Model file for the job. Use its own axes, mm. A direction names the side the tool comes from. Coordinates: 2 decimals unless noted, no trailing zeros. Write each loop counter-clockwise with the first axis right and the second up, starting at its lowest first coordinate (ties: lowest second). Pieces come first, ordered by that corner, then holes. Notation, with made-up numbers: (-15, 58) -> (13, 58) arc R25 cw to (13, 76) -> close; hole circle Ø4 at (1, 63). An arc over 180 degrees is marked (long way). Answer as a JSON object with one key per item and string values. Group by question number.
from build123d import *

# Parameters (mm, degrees)
F1_DEPTH = 63.5
F2_DEPTH = 7.9375
F3_R     = 6.35
F4_DEPTH = 25.4


with BuildPart() as f1:
    # F0 (on Front) → F1 (new body, symmetric)
    with BuildSketch(Plane.XZ):
        Polygon((22.225, 9.525), (-41.275, 9.525), (-41.275, -9.525), (41.275, -9.525), (41.275, 9.525), align=None)
    extrude(amount=F1_DEPTH, both=True)

    # F0 (on Front) → F2 (join, symmetric)
    with BuildSketch(Plane.XZ):
        with BuildLine():
            add(Edge.make_bspline(
                [(-41.275, 9.525), (-41.231316, 40.761163), (-0.825848, 60.309073), (55.42913, 61.882778)],
                knots=[0, 0, 0, 0, 110.382184, 110.382184, 110.382184, 110.382184], degree=3))
            Line((-41.275, 9.525), (22.225, 9.525))
            Line((22.225, 9.525), (22.225, 27.0002))
            ThreePointArc((22.225, 27.0002), (31.853192, 51.0798), (55.42913, 61.882778))
        make_face()
    extrude(amount=F2_DEPTH, both=True)

    # F3
    f3_edges = [f1.edges().sort_by_distance(p)[0] for p in [
        (41.275, -63.5, 0),
        (-41.275, -63.5, 0),
        (41.275, 63.5, 0),
        (-41.275, 63.5, 0),
    ]]
    fillet(f3_edges, radius=F3_R)

    # F0 (on Front) → F4 (join, symmetric)
    with BuildSketch(Plane.XZ):
        with BuildLine():
            Line((22.225, 27.0002), (22.225, 9.525))
            Line((22.225, 9.525), (41.275, 9.525))
            Line((41.275, 9.525), (41.275, 27.0002))
            ThreePointArc((41.275, 27.0002), (45.92468, 38.22552), (57.15, 42.8752))
            Line((57.15, 42.8752), (60.325, 42.8752))
            Line((60.325, 42.8752), (60.325, 61.9252))
            Line((60.325, 61.9252), (57.15, 61.9252))
            add(Edge.make_bspline(
                [(55.42913, 61.882778), (56.001123, 61.898779), (56.574755, 61.912922), (57.15, 61.9252)],
                knots=[110.382184, 110.382184, 110.382184, 110.382184, 111.504536, 111.504536, 111.504536, 111.504536], degree=3))
            ThreePointArc((55.42913, 61.882778), (31.853192, 51.0798), (22.225, 27.0002))
        make_face()
        Polygon((60.325, 66.675), (60.325, 61.9252), (60.325, 42.8752), (85.435174, 42.8752), (85.435174, 66.675), align=None)
    extrude(amount=F4_DEPTH, both=True)

    # F0 (on Front) → F5 (revolve)
    with BuildSketch(Plane.XZ):
        Polygon((85.435174, 66.675), (85.435174, 42.8752), (85.435174, 38.1), (111.125, 38.1), (111.125, 66.675), align=None)
    revolve(axis=Axis((85.435174, 0, 52.3875), (0, 0, 1)))


solid = f1.part
(1) Pin check, flat tips, straight feed: pin 1 (2.5 mm diameter, centred on y = 12, z = 65.5, fed in from -X) (3 decimals); pin 2 (10 mm diameter, centred on y = -31.5, z = 5, fed in from +X) (3 decimals); pin 3 (6 mm diameter, centred on x = 80.5, z = 37.5, fed in from +Y); pin 4 (14 mm diameter, centred on y = -16.5, z = 14.5, fed in from -X) (3 decimals). Stop position of each tip, or through.
(2) Wall check: probe 1 along Y at (x, z) = (72.5, 52); probe 2 along X at (y, z) = (48, -0.5) (3 decimals); probe 3 along Z at (x, y) = (-31, 22.5) (3 decimals). Give the ranges that are in metal, low to high.
(3) Pull direction X, two halves, no side cores. Call faces 1 (the face through (-41.275, -1, 0)), 2 (the face through (0, 63.5, 0)), 3 (the face through (59, 2, 42.875)): released by +X, released by -X, zero draft, split by the parting line, or undercut.
(4) Cut at A-A on y = 43. List the corners of the cut face in (x, z) (3 decimals).
(5) 3-axis set-ups, long thin cutter, end or side, ignore diameter. For faces 4 (the face through (86, 0, 38.1)), 5 (the face through (51, 25.4, 45)), 6 (the face through (59.745, 0.077, 64.333)), 7 (the face through (60.325, -16, 64)): which of +Z, -Z, +X, -X, +Y, -Y reach the whole face in a straight line?
Results found:
{
 "1": {"pin 1": "stops at x = 60.325", "pin 2": "stops at x = 41.275", "pin 3": "stops at y = 25.61", "pin 4": "stops at x = -41.275"},
 "2": {"probe 1": "y = -25.4 to 25.4", "probe 2": "x = -41.275 to 41.275", "probe 3": "z = -9.525 to 9.525"},
 "3": {"face 1": "released by -X", "face 2": "zero draft", "face 3": "undercut"},
 "4": {"outline": "(-41.275, -9.525) -> (41.275, -9.525) -> (41.275, 9.525) -> (-41.275, 9.525) -> close"},
 "5": {"face 4": "-Z, +X, +Y, -Y", "face 5": "+Z, -X, +Y", "face 6": "+Z, -X", "face 7": "+Z, -X, -Y"}
}
